Can you work these out from the model? Positions are in its coordinate system, mm. A direction names the side the tool comes from. Give positions to 0.01 mm unless a question says otherwise; leave off trailing zeros. Loops run counter-clockwise (first coordinate to the right, second up) from the corner with the lowest first, then second, coordinate; pieces in that order, holes last. Notation, with made-up numbers: (7, -11.5) - (44, -11.5) arc R17 ccw to (44, 11.5) - close; hole circle Ø6 at (67, 29.25). An arc over 180 degrees is marked (long way). Use a Markdown table: item, result. Add a question column.
Autodesk Fusion 360 part; units mm, degrees
sketch "Sketch1" plane through (0, 0, 0) normal (0, 0, 1) x (1, 0, 0)
  line L0 (70, 50) -> (70, -10)
  line L1 (70, -10) -> (0, -10)
  line L2 (0, -10) -> (0, 50)
  circle A0 centre (35, 50) radius 20
  arc A1 (70, 50) -> (0, 50) centre (35, 50) ccw
  line L3 (10, 5) -> (60, 5)
  line L4 (60, 5) -> (60, 20)
  line L5 (60, 20) -> (10, 20)
  line L6 (10, 20) -> (10, 5)
  dimension "d1" = 40
extrude "Extrude1" add sketch "Sketch1" along normal blind 20
1. Suppose I cut it at A-A (x = 35). List the corners of the cut face in (y, z) for me, and give its area (3 significant figures).
2. Suppose I cut it at D-D (y = 78.5). List the corners of the cut face in (x, z) for me, and give its area (3 significant figures).
3. On a 3-axis mill with a long thin cutter (end or side, diameter ignored), from which of +Z, -Z, +X, -X, +Y, -Y can I reach the whole of each face in a straight line? I mean faces 5 (the face through (35, 5, 10)), 6 (the face through (70, 20, 10)). Say none if no direction works.
4. Please list where these lines run through material, in increasing order: line 1 along Y through (x, z) = (35, 11.5); line 2 along Y through (x, z) = (29, 7); line 3 along X through (y, z) = (13, 14.75). Write a range as [from, to].
5. If we mould it in two halves opening along X, with no side actions, what happens to faces 1 (the face through (35, 28, 20)), 2 (the face through (0, 20, 10)), 3 (the face through (35, 20, 10)), 4 (the face through (54.076, 43.993, 9.86))? For each: released by +X, released by -X, zero draft, split by the parting line, or undercut.
6. Will these pins go through, and if not, where does the flat tip stop? P1, Ø12, axis at x = 52.5, y = 36, coming from the -Z side; P2, Ø2, axis at x = 57, z = 12, coming from the +Y side; P3, Ø10, axis at x = 30.5, z = 9.5, coming from the +Y side; P4, Ø1, axis at y = 61.5, z = 4.5, coming from the +X side.
7. Suppose I cut it at B-B (z = 9.75). List the corners of the cut face in (x, y) for me, and give its area (3 significant figures).
8. Suppose I cut it at C-C (x = 54). List the corners of the cut face in (y, z) for me (3 decimals), and give its area (3 significant figures).
Results below:
| question | item | result |
|---|---|---|
| 1 | outline | (-10, 0) - (5, 0) - (5, 20) - (-10, 20) - close; (20, 0) - (30, 0) - (30, 20) - (20, 20) - close; (70, 0) - (85, 0) - (85, 20) - (70, 20) - close |
| 1 | area | 800 mm² |
| 2 | outline | (14.68, 0) - (55.32, 0) - (55.32, 20) - (14.68, 20) - close |
| 2 | area | 813 mm² |
| 3 | face 5 | +Z, -Z |
| 3 | face 6 | +Z, -Z, +X, +Y, -Y |
| 4 | line 1 | [-10, 5], [20, 30], [70, 85] |
| 4 | line 2 | [-10, 5], [20, 30.92], [69.08, 84.48] |
| 4 | line 3 | [0, 10], [60, 70] |
| 5 | face 1 | zero draft |
| 5 | face 2 | released by -X |
| 5 | face 3 | undercut |
| 5 | face 4 | undercut |
| 6 | P1 | z = 0 |
| 6 | P2 | y = 78 |
| 6 | P3 | y = 85 |
| 6 | P4 | x = 68.23 |
| 7 | outline | (0, -10) - (70, -10) - (70, 50) arc R35 ccw to (0, 50) - close; hole (10, 5) - (60, 5) - (60, 20) - (10, 20) - close; hole circle Ø40 at (35, 50) |
| 7 | area | 4,120 mm² |
| 8 | outline | (-10, 0) - (5, 0) - (5, 20) - (-10, 20) - close; (20, 0) - (43.755, 0) - (43.755, 20) - (20, 20) - close; (56.245, 0) - (79.394, 0) - (79.394, 20) - (56.245, 20) - close |
| 8 | area | 1,240 mm² |
